Verification items for the finished model (mm, model axes). Give positions to 0.01 mm unless a question says otherwise; leave off trailing zeros. Loops run counter-clockwise (first coordinate to the right, second up) from the corner with the lowest first, then second, coordinate; pieces in that order, holes last. Notation, with made-up numbers: (-26, 81) - (6, 81) arc R26 ccw to (6, 100) - close; hole circle Ø6 at (-24.5, 69). An arc over 180 degrees is marked (long way). One line per question, with ' | ' between items. Start each with the question number.
1. Section check A-A, the plane y = 0. Enter the section's corners in (x, z), then the cut area to 3 significant figures.
2. Thickness scan on line 1 along Z through (x, y) = (15, 4.5); line 2 along X through (y, z) = (2.5, 60); line 3 along Y through (x, z) = (-26, 61.5). Record the ranges inside material, lowest first. Write a range as from..to.
3. Section check C-C, the plane x = -11. Enter the section's corners in (y, z), then the cut area to 3 significant figures.
4. Section check D-D, the plane x = 14. Enter the section's corners in (y, z).
5. Depth check by flat-ended pin: pin 1 Ø3 at (x, y) = (3, -9) entering from +Z; pin 2 Ø6 at (y, z) = (-5, 65) entering from -X; pin 3 Ø8 at (y, z) = (-4, 59.5) entering from -X. Enter the tip coordinate at first touch or a pass-through.
6. Mould release check, pull along X, two halves, no side actions. Record for faces 1 (the face through (-37.861, 1, 24)), 2 (the face through (2, -31.797, 24)), 3 (the face through (-31.27, 0.19, 61.12)), 4 (the face through (-6.317, -2.35, 61.125)): +X half, -X half, draft (parallel to the pull), parting line (faces both ways), or undercut.
7. Section check B-B, the plane z = 52.5. Enter the section's corners in (x, y).
from build123d import *

# Parameters (mm, degrees)
F0_W     = 80.157895
F0_H     = 67.439113
F1_DEPTH = 48.8
F2_W     = 64.96834
F2_H     = 55.503204
F3_DEPTH = 20
F4_R     = 4.292628
F5_DEPTH = 25
F6_R     = 6.135078
F7_DEPTH = 25


with BuildPart() as f1:
    # F0 (on Top) → F1 (new body)
    with BuildSketch(Plane.XY):
        with Locations((2.218393, 1.922605)):
            Rectangle(F0_W, F0_H)
    extrude(amount=F1_DEPTH)

    # F2 (on face) → F3 (join)
    with BuildSketch(Plane.XY.offset(48.8)):
        with Locations((3.307585, 3.803581)):
            Rectangle(F2_W, F2_H)
    extrude(amount=-F3_DEPTH)

    # F4 (on face) → F5 (join)
    with BuildSketch(Plane.XY.offset(48.8)):
        with Locations((-26.979957, 0)):
            Circle(F4_R)
    extrude(amount=F5_DEPTH)

    # F6 (on face) → F7 (join)
    with BuildSketch(Plane.XY.offset(48.8)):
        with Locations((-11.984075, 0)):
            Circle(F6_R)
    extrude(amount=F7_DEPTH)


solid = f1.part
Results list:
1) outline: (-37.86, 0) - (42.3, 0) - (42.3, 48.8) - (-5.85, 48.8) - (-5.85, 73.8) - (-18.12, 73.8) - (-18.12, 48.8) - (-22.69, 48.8) - (-22.69, 73.8) - (-31.27, 73.8) - (-31.27, 48.8) - (-37.86, 48.8) - close | area: 4,430 mm²
2) line 1: 0..48.8 | line 2: -30.47..-23.49, -17.59..-6.38 | line 3: -4.18..4.18
3) outline: (-31.8, 0) - (35.64, 0) - (35.64, 48.8) - (6.06, 48.8) - (6.06, 73.8) - (-6.06, 73.8) - (-6.06, 48.8) - (-31.8, 48.8) - close | area: 3,590 mm²
4) outline: (-31.8, 0) - (35.64, 0) - (35.64, 48.8) - (-31.8, 48.8) - close
5) pin 1: z = 48.8 | pin 2: x = -30.78 | pin 3: x = -31.27
6) face 1: -X half | face 2: draft | face 3: undercut | face 4: undercut
7) outline: circle Ø8.59 at (-26.98, 0); circle Ø12.27 at (-11.98, 0)
